```python
from build123d import *

# Parameters (mm, degrees)
F0_W     = 101.6
F0_H     = 31.75
F1_DEPTH = 31.75
F2_T     = -1.5875
F4_D     = 9.525
F5_ANGLE = 90
F6_ANGLE = 180


with BuildPart() as f1:
    # F0 (on Top) → F1 (new body)
    with BuildSketch(Plane.XY):
        with Locations((-50.8, 15.875)):
            Rectangle(F0_W, F0_H)
    extrude(amount=F1_DEPTH)

    # F2
    f2_openings = [f1.faces().sort_by_distance(p)[0] for p in [
        (-101.6, 15.875, 15.875),
        (0, 15.875, 15.875),
    ]]
    offset(amount=F2_T, openings=f2_openings)

    # F4 (through all)
    with Locations(Plane.XY.offset(31.75)):
        with Locations((-35.8643569052, 16.9158093631)):
            Hole(F4_D / 2)


with BuildPart() as f1_1:
    # F5: moved
    add(f1.part.rotate(Axis((-50.8, 31.75, 31.75), (-1, 0, 0)), F5_ANGLE))


with BuildPart() as f1_2:
    # F6: moved
    add(f1_1.part.rotate(Axis((-101.6, 0, 47.625), (0, 0, -1)), F6_ANGLE))


solid = f1_2.part
```
Can you work these out from the model? Positions are in its coordinate system, mm. A direction names the side the tool comes from. Give positions to 0.01 mm unless a question says otherwise; leave off trailing zeros. Write each loop counter-clockwise with the first axis right and the second up, starting at its lowest first coordinate (ties: lowest second). Pieces come first, ordered by that corner, then holes. Notation, with made-up numbers: (10, 0) -> (22, 0) arc R22 ccw to (22, 21) -> close; hole circle Ø2 at (-13, 49.5). An arc over 180 degrees is marked (long way). Write item = value, one per line.
(1) For faces 1 (the face through (-152, -16, 33.338)), 2 (the face through (-162.936, -30.945, 48.408)), which set-ups out of +Z, -Z, +X, -X, +Y, -Y let a thin tool reach every point of the face, with its end or its side?
Worked out:
face_1 = +X, -X
face_2 = +Y, -Y
(2) Thinking about a two-plate mould opening in Z: for faces 3 (the face through (-152, -16, 31.75)), 4 (the face through (-162.936, -0.783, 48.408)), 5 (the face through (-203.2, -31, 49)), 6 (the face through (-152, -16, 63.5)), which applies, released by +Z, released by -Z, zero draft, split by the parting line, or undercut?
Worked out:
face_3 = released by -Z
face_4 = undercut
face_5 = zero draft
face_6 = released by +Z
(3) Suppose I cut it at A-A on y = -7. Write out the boundary of the cut face in (x, z).
Worked out:
outline = (-203.2, 31.75) -> (-101.6, 31.75) -> (-101.6, 33.34) -> (-203.2, 33.34) -> close; (-203.2, 61.91) -> (-101.6, 61.91) -> (-101.6, 63.5) -> (-203.2, 63.5) -> close
(4) I need wall thicknesses on probe 1 along Z at (x, y) = (-125.5, -14); probe 2 along Y at (x, z) = (-118, 34.5). Which ranges of each line are inside material? Lowest first, please. Write a range as from..to.
Worked out:
probe_1 = 31.75..33.34, 61.91..63.5
probe_2 = -31.75..-30.16, -1.59..0
(5) Suppose I cut it at B-B on z = 39.5. Write out the boundary of the cut face in (x, y), then the cut area to 3 significant figures.
Worked out:
outline = (-203.2, -31.75) -> (-101.6, -31.75) -> (-101.6, -30.16) -> (-203.2, -30.16) -> close; (-203.2, -1.59) -> (-101.6, -1.59) -> (-101.6, 0) -> (-203.2, 0) -> close
area = 323 mm^2
(6) Suppose I cut it at D-D on z = 50. Write out the boundary of the cut face in (x, y).
Worked out:
outline = (-203.2, -31.75) -> (-170.65, -31.75) -> (-170.65, -30.16) -> (-203.2, -30.16) -> close; (-203.2, -1.59) -> (-170.65, -1.59) -> (-170.65, 0) -> (-203.2, 0) -> close; (-164.02, -31.75) -> (-101.6, -31.75) -> (-101.6, -30.16) -> (-164.02, -30.16) -> close; (-164.02, -1.59) -> (-101.6, -1.59) -> (-101.6, 0) -> (-164.02, 0) -> close
(7) Suppose I cut it at C-C on x = -173.5. Write out the boundary of the cut face in (y, z).
Worked out:
outline = (-31.75, 31.75) -> (0, 31.75) -> (0, 63.5) -> (-31.75, 63.5) -> close; hole (-30.16, 33.34) -> (-1.59, 33.34) -> (-1.59, 61.91) -> (-30.16, 61.91) -> close
